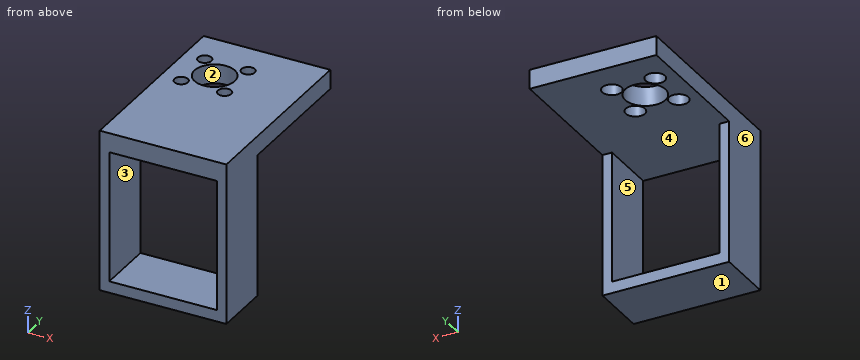
```python
from build123d import *

# Parameters (mm, degrees)
SZKIC1_W                    = 33
SZKIC1_H                    = 15
DODANIE_WYCI_GNI_CIE1_DEPTH = 40
SZKIC2_W                    = 28
SZKIC2_H                    = 34
WYTNIJ_WYCI_GNI_CIE1_DEPTH  = 29
SZKIC3_W                    = 33
SZKIC3_H                    = 50
DODANIE_WYCI_GNI_CIE2_DEPTH = 2
SZKIC3_3_R                  = 4
WYTNIJ_WYCI_GNI_CIE2_DEPTH  = 16
SZKIC7_W                    = 33
SZKIC7_H                    = 50
DODANIE_WYCI_GNI_CIE3_DEPTH = 3
SZKIC3_5_R                  = 1.75
WYTNIJ_WYCI_GNI_CIE5_DEPTH  = 14.5
SZKIC3_6_R                  = 1.75
WYTNIJ_WYCI_GNI_CIE6_DEPTH  = 14.5
SZKIC3_7_R                  = 1.75
WYTNIJ_WYCI_GNI_CIE7_DEPTH  = 8.5
SZKIC5_R                    = 5.25
WYTNIJ_WYCI_GNI_CIE10_DEPTH = 36
SZKIC3_8_R                  = 1.75
WYTNIJ_WYCI_GNI_CIE8_DEPTH  = 5.5
SZKIC9_R                    = 2.5
WYTNIJ_WYCI_GNI_CIE11_DEPTH = 3
SZKIC9_4_R                  = 2.5
WYTNIJ_WYCI_GNI_CIE12_DEPTH = 3
SZKIC9_5_R                  = 2.5
WYTNIJ_WYCI_GNI_CIE13_DEPTH = 3
SZKIC9_6_R                  = 2.5
WYTNIJ_WYCI_GNI_CIE14_DEPTH = 3


with BuildPart() as part:
    # Szkic1 → Dodanie-wyci_gni_cie1 (new body)
    with BuildSketch(Plane.XY):
        Rectangle(SZKIC1_W, SZKIC1_H)
    extrude(amount=DODANIE_WYCI_GNI_CIE1_DEPTH)

    # Szkic2 → Wytnij-wyci_gni_cie1 (cut)
    with BuildSketch(Plane(origin=(0, 7.5, 0), x_dir=(1, 0, 0), z_dir=(0, 1, 0))):
        with Locations((0, -20)):
            Rectangle(SZKIC2_W, SZKIC2_H)
    extrude(amount=-WYTNIJ_WYCI_GNI_CIE1_DEPTH, mode=Mode.SUBTRACT)

    # Szkic3 → Dodanie-wyci_gni_cie2 (add)
    with BuildSketch(Plane.XY.offset(40)):
        with Locations((0, 17.5)):
            Rectangle(SZKIC3_W, SZKIC3_H)
    extrude(amount=DODANIE_WYCI_GNI_CIE2_DEPTH)

    # Szkic3_3 → Wytnij-wyci_gni_cie2 (cut)
    with BuildSketch(Plane.XY.offset(40)):
        with Locations(Location((-5.5, 27.5, 0), (0, 0, 180))):
            Circle(SZKIC3_3_R)
    extrude(amount=WYTNIJ_WYCI_GNI_CIE2_DEPTH, mode=Mode.SUBTRACT)

    # Szkic7 → Dodanie-wyci_gni_cie3 (add)
    with BuildSketch(Plane(origin=(0, 0, 40), x_dir=(-1, 0, 0), z_dir=(0, 0, -1))):
        with Locations((0, 17.5)):
            Rectangle(SZKIC7_W, SZKIC7_H)
    extrude(amount=DODANIE_WYCI_GNI_CIE3_DEPTH)

    # Szkic3_5 → Wytnij-wyci_gni_cie5 (cut, symmetric)
    with BuildSketch(Plane.XY.offset(40)):
        with Locations(Location((-11.156854249, 33.156854249, 0), (0, 0, 180))):
            Circle(SZKIC3_5_R)
    extrude(amount=WYTNIJ_WYCI_GNI_CIE5_DEPTH, both=True, mode=Mode.SUBTRACT)

    # Szkic3_6 → Wytnij-wyci_gni_cie6 (cut, symmetric)
    with BuildSketch(Plane.XY.offset(40)):
        with Locations(Location((-11.156854249, 21.843145751, 0), (0, 0, 180))):
            Circle(SZKIC3_6_R)
    extrude(amount=WYTNIJ_WYCI_GNI_CIE6_DEPTH, both=True, mode=Mode.SUBTRACT)

    # Szkic3_7 → Wytnij-wyci_gni_cie7 (cut, symmetric)
    with BuildSketch(Plane.XY.offset(40)):
        with Locations(Location((0.156854249, 33.156854249, 0), (0, 0, 180))):
            Circle(SZKIC3_7_R)
    extrude(amount=WYTNIJ_WYCI_GNI_CIE7_DEPTH, both=True, mode=Mode.SUBTRACT)

    # Szkic5 → Wytnij-wyci_gni_cie10 (cut)
    with BuildSketch(Plane.XY.offset(42)):
        with Locations((-5.5, 27.5)):
            Circle(SZKIC5_R)
    extrude(amount=-WYTNIJ_WYCI_GNI_CIE10_DEPTH, mode=Mode.SUBTRACT)

    # Szkic3_8 → Wytnij-wyci_gni_cie8 (cut, symmetric)
    with BuildSketch(Plane.XY.offset(40)):
        with Locations(Location((0.156854249, 21.843145751, 0), (0, 0, 180))):
            Circle(SZKIC3_8_R)
    extrude(amount=WYTNIJ_WYCI_GNI_CIE8_DEPTH, both=True, mode=Mode.SUBTRACT)

    # Szkic9 → Wytnij-wyci_gni_cie11 (cut)
    with BuildSketch(Plane(origin=(0, 0, 37), x_dir=(-1, 0, 0), z_dir=(0, 0, -1))):
        with Locations((-0.156854249, 33.156854249)):
            Circle(SZKIC9_R)
    extrude(amount=-WYTNIJ_WYCI_GNI_CIE11_DEPTH, mode=Mode.SUBTRACT)

    # Szkic9_4 → Wytnij-wyci_gni_cie12 (cut)
    with BuildSketch(Plane(origin=(0, 0, 37), x_dir=(-1, 0, 0), z_dir=(0, 0, -1))):
        with Locations((11.156854249, 33.156854249)):
            Circle(SZKIC9_4_R)
    extrude(amount=-WYTNIJ_WYCI_GNI_CIE12_DEPTH, mode=Mode.SUBTRACT)

    # Szkic9_5 → Wytnij-wyci_gni_cie13 (cut)
    with BuildSketch(Plane(origin=(0, 0, 37), x_dir=(-1, 0, 0), z_dir=(0, 0, -1))):
        with Locations((11.156854249, 21.843145751)):
            Circle(SZKIC9_5_R)
    extrude(amount=-WYTNIJ_WYCI_GNI_CIE13_DEPTH, mode=Mode.SUBTRACT)

    # Szkic9_6 → Wytnij-wyci_gni_cie14 (cut)
    with BuildSketch(Plane(origin=(0, 0, 37), x_dir=(-1, 0, 0), z_dir=(0, 0, -1))):
        with Locations((-0.156854249, 21.843145751)):
            Circle(SZKIC9_6_R)
    extrude(amount=-WYTNIJ_WYCI_GNI_CIE14_DEPTH, mode=Mode.SUBTRACT)


solid = part.part
```
Build history of the part. All positions in model axes, mm. Face numbers are marked on the shaded views. A direction names the side the tool comes from. Give positions to 0.01 mm unless a question says otherwise; leave off trailing zeros. Loops run counter-clockwise (first coordinate to the right, second up) from the corner with the lowest first, then second, coordinate; pieces in that order, holes last. Notation, with made-up numbers: (72, 44) - (115, 44) arc R21 ccw to (115, 79) - close; hole circle Ø9 at (65.25, 45). An arc over 180 degrees is marked (long way). Use a Markdown table: item, result.
(1) Band-saw the part on B-B (y = 27.5). Give the cut face in (x, z), and give its area (4 significant figures).
Taken from the geometry:
| item | result |
|---|---|
| outline | (-16.5, 37) - (-10.75, 37) - (-10.75, 42) - (-16.5, 42) - close; (-0.25, 37) - (16.5, 37) - (16.5, 42) - (-0.25, 42) - close |
| area | 112.5 mm2 |
(2) Band-saw the part on C-C (z = 32.5). Give the cut face in (x, y), and give its area (3 significant figures).
Taken from the geometry:
| item | result |
|---|---|
| outline | (-16.5, -7.5) - (-14, -7.5) - (-14, 7.5) - (-16.5, 7.5) - close; (14, -7.5) - (16.5, -7.5) - (16.5, 7.5) - (14, 7.5) - close |
| area | 75.0 mm2 |
(3) Drop flat-ended pins along their axis: pin 1 Ø4 at (x, y) = (-10, 23) entering from -Z; pin 2 Ø8 at (x, z) = (-12, 18.5) entering from -Y; pin 3 Ø16.5 at (x, z) = (-4.5, 18) entering from +Y; pin 4 Ø1.5 at (x, y) = (1.5, 21.5) entering from -Z. Give the stop position or say it passes through.
Taken from the geometry:
| item | result |
|---|---|
| pin 1 | z = 37 |
| pin 2 | y = -7.5 |
| pin 3 | through |
| pin 4 | z = 40 |
(4) Pull direction Z, two halves, no side cores. Call the marked faces 1, 2 and 3: +Z half, -Z half, draft (parallel to the pull), parting line (faces both ways), or undercut.
Taken from the geometry:
| item | result |
|---|---|
| face 1 | -Z half |
| face 2 | draft |
| face 3 | undercut |
(5) Wall check: line 1 along X through (y, z) = (5.5, 9); line 2 along Z through (x, y) = (-9, -0.5); line 3 along Y through (x, z) = (-12, 38.5). Give the ranges that are in metal, low to high.
Taken from the geometry:
| item | result |
|---|---|
| line 1 | -16.5 to -14, 14 to 16.5 |
| line 2 | 0 to 3, 37 to 42 |
| line 3 | -7.5 to 19.49, 24.2 to 30.8, 35.51 to 42.5 |
(6) Band-saw the part on D-D (y = 1.5). Give the cut face in (x, z), and give its area (3 significant figures).
Taken from the geometry:
| item | result |
|---|---|
| outline | (-16.5, 0) - (16.5, 0) - (16.5, 42) - (-16.5, 42) - close; hole (-14, 3) - (14, 3) - (14, 37) - (-14, 37) - close |
| area | 434 mm2 |
(7) Band-saw the part on A-A (x = -5.5). Give the cut face in (y, z).
Taken from the geometry:
| item | result |
|---|---|
| outline | (-7.5, 0) - (7.5, 0) - (7.5, 3) - (-7.5, 3) - close; (-7.5, 37) - (22.25, 37) - (22.25, 42) - (-7.5, 42) - close; (32.75, 37) - (42.5, 37) - (42.5, 42) - (32.75, 42) - close |
(8) Which spindle directions (+Z, -Z, +X, -X, +Y, -Y) get a long thin tool onto all of the face, cutting with end or side? Do the marked faces 4, 5 and 6. Say none if no direction does.
Taken from the geometry:
| item | result |
|---|---|
| face 4 | +Y |
| face 5 | +Y, -Y |
| face 6 | +Z, -Z, -X, +Y, -Y |
